Geometry check sheet. Reference: the model listing, model coordinates, mm. A direction names the side the tool comes from. Coordinates: 2 decimals unless noted, no trailing zeros. Write each loop counter-clockwise with the first axis right and the second up, starting at its lowest first coordinate (ties: lowest second). Pieces come first, ordered by that corner, then holes.
from build123d import *

# Parameters (mm, degrees)
SKETCH1_R           = 50
BOSS_EXTRUDE1_DEPTH = 2
SKETCH2_R           = 48
SKETCH2_R_2         = 47
BOSS_EXTRUDE2_DEPTH = 4
BOSS_EXTRUDE3_START = -2
SKETCH3_R           = 2.5
BOSS_EXTRUDE3_DEPTH = 2


with BuildPart() as part:
    # Sketch1 → Boss-Extrude1 (new body)
    with BuildSketch(Plane(origin=(0, 0, 0), x_dir=(1, 0, 0), z_dir=(0, 1, 0))):
        with Locations(Location((0, 0, 0), (0, 0, 270))):
            Circle(SKETCH1_R)
    extrude(amount=BOSS_EXTRUDE1_DEPTH)

    # Sketch2 → Boss-Extrude2 (add)
    with BuildSketch(Plane(origin=(0, 2, 0), x_dir=(1, 0, 0), z_dir=(0, 1, 0))):
        with Locations(Location((0, 0, 0), (0, 0, 270))):
            Circle(SKETCH2_R)
        with Locations(Location((0, 0, 0), (0, 0, 270))):
            Circle(SKETCH2_R_2, mode=Mode.SUBTRACT)
    extrude(amount=BOSS_EXTRUDE2_DEPTH)

    # Sketch3 → Boss-Extrude3 (add)
    # profile 1 of 4: a face of its own
    with BuildSketch(Plane(origin=(0, 2, 0), x_dir=(1, 0, 0), z_dir=(0, 1, 0)).offset(BOSS_EXTRUDE3_START)):
        with BuildLine():
            Line((-55.759371855, 5), (-49.749371855, 5))
            ThreePointArc((-49.749371855, 5), (-50, 0), (-49.749371855, -5))
            Line((-49.749371855, -5), (-55.759371855, -5))
            ThreePointArc((-55.759371855, -5), (-59.380980039, -3.54948202), (-61, 0))
            ThreePointArc((-61, 0), (-59.380980039, 3.54948202), (-55.759371855, 5))
        make_face()
        with Locations(Location((-56, 0, 0), (0, 0, 270))):
            Circle(SKETCH3_R, mode=Mode.SUBTRACT)
    # profile 2 of 4: a face of its own
    with BuildSketch(Plane(origin=(0, 2, 0), x_dir=(1, 0, 0), z_dir=(0, 1, 0)).offset(BOSS_EXTRUDE3_START)):
        with BuildLine():
            Line((5, 55.759371855), (5, 49.749371855))
            ThreePointArc((5, 49.749371855), (0, 50), (-5, 49.749371855))
            Line((-5, 49.749371855), (-5, 55.759371855))
            ThreePointArc((-5, 55.759371855), (-3.54948202, 59.380980039), (0, 61))
            ThreePointArc((0, 61), (3.54948202, 59.380980039), (5, 55.759371855))
        make_face()
        with Locations(Location((0, 56, 0), (0, 0, 270))):
            Circle(SKETCH3_R, mode=Mode.SUBTRACT)
    # profile 3 of 4: a face of its own
    with BuildSketch(Plane(origin=(0, 2, 0), x_dir=(1, 0, 0), z_dir=(0, 1, 0)).offset(BOSS_EXTRUDE3_START)):
        with BuildLine():
            Line((55.759371855, -5), (49.749371855, -5))
            ThreePointArc((49.749371855, -5), (50, 0), (49.749371855, 5))
            Line((49.749371855, 5), (55.759371855, 5))
            ThreePointArc((55.759371855, 5), (59.380980039, 3.54948202), (61, 0))
            ThreePointArc((61, 0), (59.380980039, -3.54948202), (55.759371855, -5))
        make_face()
        with Locations(Location((56, 0, 0), (0, 0, 270))):
            Circle(SKETCH3_R, mode=Mode.SUBTRACT)
    # profile 4 of 4: a face of its own
    with BuildSketch(Plane(origin=(0, 2, 0), x_dir=(1, 0, 0), z_dir=(0, 1, 0)).offset(BOSS_EXTRUDE3_START)):
        with BuildLine():
            Line((-5, -55.759371855), (-5, -49.749371855))
            ThreePointArc((-5, -49.749371855), (0, -50), (5, -49.749371855))
            Line((5, -49.749371855), (5, -55.759371855))
            ThreePointArc((5, -55.759371855), (3.54948202, -59.380980039), (0, -61))
            ThreePointArc((0, -61), (-3.54948202, -59.380980039), (-5, -55.759371855))
        make_face()
        with Locations(Location((0, -56, 0), (0, 0, 270))):
            Circle(SKETCH3_R, mode=Mode.SUBTRACT)
    extrude(amount=BOSS_EXTRUDE3_DEPTH)


solid = part.part
1. Thickness scan on line 1 along X through (y, z) = (1.1, 56); line 2 along Y through (x, z) = (-26.5, 14); line 3 along X through (y, z) = (3.8, -35). Record the ranges inside material, lowest first.
Computed values:
line 1: x = -4.99 to -2.5, 2.5 to 4.99
line 2: y = 0 to 2
line 3: x = -32.85 to -31.37, 31.37 to 32.85
2. Gauge pin test, flat ends, axial feed: pin 1 Ø1.5 at (y, z) = (0.5, 46) entering from -X; pin 2 Ø6.5 at (x, z) = (-56, 0) entering from +Y; pin 3 Ø1 at (y, z) = (1, -53) entering from +X; pin 4 Ø4 at (x, z) = (0, -56) entering from -Y. Record the tip position at first contact, or that the pin passes through.
Computed values:
pin 1: stops at x = -21.27
pin 2: stops at y = 2
pin 3: stops at x = 5
pin 4: passes through
3. Sectioned sample at A-A, the plane y = 1. Record the boundary of the cut face in (x, z).
Computed values:
outline: (-61, 0) arc R5.25 ccw to (-55.76, -5) - (-49.75, -5) arc R50 ccw to (-5, -49.75) - (-5, -55.76) arc R5.25 ccw to (0, -61) arc R5.25 ccw to (5, -55.76) - (5, -49.75) arc R50 ccw to (49.75, -5) - (55.76, -5) arc R5.25 ccw to (61, 0) arc R5.25 ccw to (55.76, 5) - (49.75, 5) arc R50 ccw to (5, 49.75) - (5, 55.76) arc R5.25 ccw to (0, 61) arc R5.25 ccw to (-5, 55.76) - (-5, 49.75) arc R50 ccw to (-49.75, 5) - (-55.76, 5) arc R5.25 ccw to start; hole circle Ø5 at (-56, 0); hole circle Ø5 at (0, -56); hole circle Ø5 at (0, 56); hole circle Ø5 at (56, 0)
4. Draft check along Z on faces 1 (the cylindrical face through (-35.693, 0.986, 35.015)), 2 (the cylindrical face through (-59.42, 0.99, -3.51)), 3 (the cylindrical face through (-0.96, 0.99, -53.69)), 4 (the cylindrical face through (14.418, 3.972, 45.783)). Enter one of: released by +Z, released by -Z, zero draft, split by the parting line, or undercut.
Computed values:
face 1: released by +Z
face 2: released by -Z
face 3: undercut
face 4: split by the parting line
5. Sectioned sample at B-B, the plane z = -10.5. Record the boundary of the cut face in (x, y), and give its area (3 significant figures).
Computed values:
outline: (-48.89, 0) - (48.89, 0) - (48.89, 2) - (46.84, 2) - (46.84, 6) - (45.81, 6) - (45.81, 2) - (-45.81, 2) - (-45.81, 6) - (-46.84, 6) - (-46.84, 2) - (-48.89, 2) - close
area: 204 mm2
6. Sectioned sample at C-C, the plane z = -40. Record the boundary of the cut face in (x, y), and give its area (3 significant figures).
Computed values:
outline: (-30, 0) - (30, 0) - (30, 2) - (26.53, 2) - (26.53, 6) - (24.68, 6) - (24.68, 2) - (-24.68, 2) - (-24.68, 6) - (-26.53, 6) - (-26.53, 2) - (-30, 2) - close
area: 135 mm2
7. Access from +Z, -Z, +X, -X, +Y, -Y to the whole of each face (thin tool, end or side, straight path). Record for faces 5 (the flat face through (1, 2, -1)), 6 (the flat face through (1, 0, -1)).
Computed values:
face 5: +Y
face 6: +Z, -Z, +X, -X, -Y
